from build123d import *

# Parameters (mm, degrees)
F1_DEPTH = 17.4625
F3_D     = 9.525
F4_R     = 6.35


with BuildPart() as f1:
    # F0 (on Top) → F1 (new body)
    with BuildSketch(Plane.XY):
        Polygon((62.708709, 41.755856), (-64.291291, 41.755856), (-64.291291, -9.044144), (-45.354009, -9.044144), (-45.354009, -28.094144), (43.545991, -28.094144), (43.545991, -9.044144), (62.708709, -9.044144), align=None)
    extrude(amount=F1_DEPTH)

    # F3 (through all)
    with Locations(Plane(origin=(-45.354009, 0, 0), x_dir=(0, -1, 0), z_dir=(-1, 0, 0))):
        with Locations((18.569144, 8.73125)):
            Hole(F3_D / 2)

    # F4
    f4_edges = [f1.edges().sort_by_distance(p)[0] for p in [
        (-0.904009, -28.094144, 17.4625),
        (-0.904009, -28.094144, 0),
    ]]
    fillet(f4_edges, radius=F4_R)


solid = f1.part
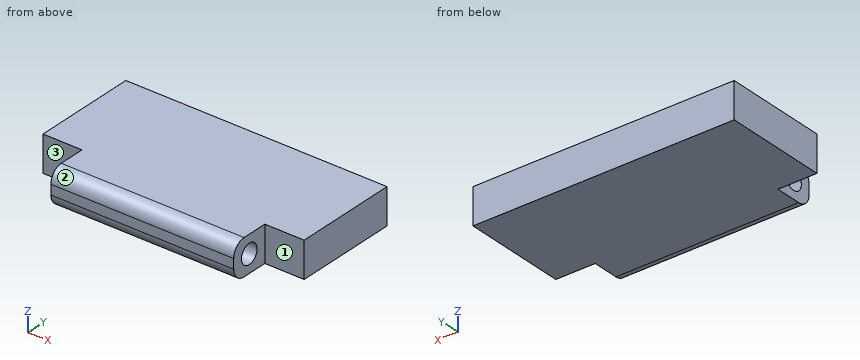
The listing builds one solid part. Answer for the finished solid, in the listing's coordinates (mm). Face numbers are marked on the shaded views. A direction names the side the tool comes from. Round coordinates to 2 decimals unless told otherwise and drop trailing zeros. Order: outer loops, then holes, each group sorted by start corner. A loop starts at its lowest first (then second) coordinate and runs counter-clockwise, first axis right, second up. Notation, with made-up numbers: (30.5, 38.25) -> (47.5, 38.25) arc R28 ccw to (47.5, 59.25) -> close; hole circle Ø7 at (9, 77.25). An arc over 180 degrees is marked (long way). Put each result on its own line as item: value.
Q1. Section D-D, the plane x = 49.5 is taken. Write down the section's boundary in (y, z).
Results list:
outline: (-9.04, 0) -> (41.76, 0) -> (41.76, 17.46) -> (-9.04, 17.46) -> close
Q2. Section C-C, the plane z = 2.25 is taken. Write down the section's boundary in (x, y), and give its area (3 significant figures).
Results list:
outline: (-64.29, -9.04) -> (-45.35, -9.04) -> (-45.35, -26.59) -> (43.55, -26.59) -> (43.55, -9.04) -> (62.71, -9.04) -> (62.71, 41.76) -> (-64.29, 41.76) -> close
area: 8,010 mm^2
Q3. Each of these flat-tipped pins is pushed along its axis until it touches: P1, Ø8.5, axis at y = -18.57, z = 8.73, coming from the -X side; P2, Ø5, axis at x = 50, z = 8.5, coming from the -Y side; P3, Ø10, axis at x = 35.5, z = 12.5, coming from the -Y side. Where does it stop, or does it pass through?
Results list:
P1: through
P2: y = -9.04
P3: y = -28.09
Q4. Section A-A, the plane y = -20.5 is taken. Write down the section's boundary in (x, z).
Results list:
outline: (-45.35, 0) -> (43.55, 0) -> (43.55, 4.38) -> (-45.35, 4.38) -> close; (-45.35, 13.08) -> (43.55, 13.08) -> (43.55, 17.46) -> (-45.35, 17.46) -> close
Q5. Consider line 1 along Y through (x, z) = (2, 9); line 2 along X through (y, z) = (-12.5, 16); line 3 along Z through (x, y) = (-9.5, -19). Determine where each line is inside the solid, lowest interval first.
Results list:
line 1: -28.09 to -23.32, -13.81 to 41.76
line 2: -45.35 to 43.55
line 3: 0 to 3.99, 13.47 to 17.46
Q6. Which of the six approach directions +Z, -Z, +X, -X, +Y, -Y give full straight-line access (tool end or side, diameter ignored) to the marked faces 1, 2 and 3?
Results list:
face 1: +Z, -Z, +X, -Y
face 2: +Z, +X, -X, -Y
face 3: +Z, -Z, -X, -Y
